from build123d import *

# Parameters (mm, degrees)
SKETCH2_R           = 0.26475865
BOSS_EXTRUDE1_DEPTH = 6.35


with BuildPart() as part:
    # Sketch1 → Revolve6 (revolve)
    with BuildSketch(Plane(origin=(0, 0, 0), x_dir=(0, 0, -1), z_dir=(1, 0, 0)), mode=Mode.PRIVATE) as revolve6_sk:
        with BuildLine():
            ThreePointArc((2.5, 0), (1.767766953, 1.767766953), (0, 2.5))
            Line((0, 2.5), (0, -7.09))
            Line((0, -7.09), (2.95, -7.09))
            Line((2.95, -7.09), (2.95, -6.09))
            Line((2.95, -6.09), (2.5, -6.09))
            Line((2.5, -6.09), (2.5, 0))
        make_face()
    revolve(revolve6_sk.sketch.rotate(Axis((0, 2.5, 0), (0, -1, 0)), 180), axis=Axis((0, 2.5, 0), (0, -1, 0)))

    # Sketch2 → Boss-Extrude1 (add)
    with BuildSketch(Plane.XZ.offset(7.09)):
        with Locations(Location((0, 1.283330706, 0), (0, 0, 90))):
            Circle(SKETCH2_R)
        with Locations(Location((0, -1.188269173, 0), (0, 0, 90))):
            Circle(SKETCH2_R)
    extrude(amount=BOSS_EXTRUDE1_DEPTH)


solid = part.part
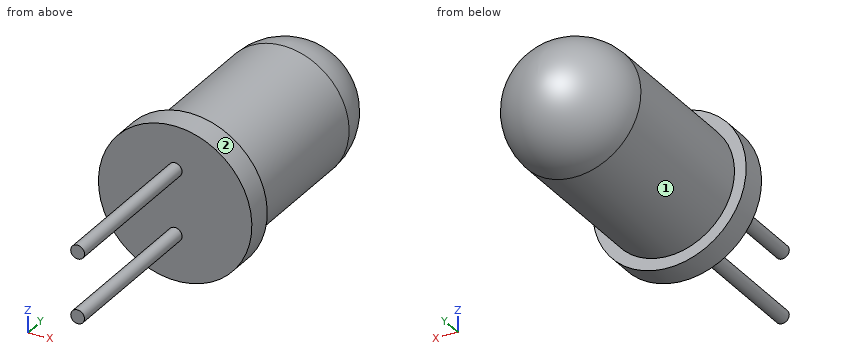
Geometry: final body of the model. Coordinates: model frame, mm. Face numbers are marked on the shaded views. A direction names the side the tool comes from. Coordinates: 2 decimals unless noted, no trailing zeros. Order: outer loops, then holes, each group sorted by start corner. A loop starts at its lowest first (then second) coordinate and runs counter-clockwise, first axis right, second up.
(1) Access query for the marked faces 1 and 2. Directions: +Z, -Z, +X, -X, +Y, -Y. A direction counts if a zero-diameter tool reaches every point of the face in a straight line with its end or side. Return the directions, or none.
(2) Material intervals for probe 1 along Y at (x, z) = (-1, -2.7); probe 2 along Z at (x, y) = (-1.7, -4.75); probe 3 along X at (y, z) = (0, -0.65), sorted ascending.
(3) Section query C-C (x = 0). Return the cut outline in (y, z).
(4) Section query D-D (y = -2). Return the cut outline in (x, z).
(5) First-contact query: pin 1 (2 mm diameter, centred on x = -2, z = 1, fed in from -Y); pin 2 (3 mm diameter, centred on x = 1, z = 0, fed in from +Y); pin 3 (3 mm diameter, centred on x = 1.5, y = 0, fed in from -Z). Flat tips, straight axial feed; report the tip coordinate or a pass-through.
(6) Section query B-B (y = -8.5). Return the cut outline in (x, z), plus the area to 3 significant figures.
(7) Section query A-A (z = 0). Return the cut outline in (x, y), plus the area to 3 significant figures.
Solution:
1. face 1: +Y
1. face 2: +Y, -Y
2. probe 1: y = -7.09 to -6.09
2. probe 2: z = -1.83 to 1.83
2. probe 3: x = -2.41 to 2.41
3. outline: (-13.44, -1.45) - (-7.09, -1.45) - (-7.09, -2.95) - (-6.09, -2.95) - (-6.09, -2.5) - (0, -2.5) arc R2.5 ccw to (0, 2.5) - (-6.09, 2.5) - (-6.09, 2.95) - (-7.09, 2.95) - (-7.09, 1.55) - (-13.44, 1.55) - (-13.44, 1.02) - (-7.09, 1.02) - (-7.09, -0.92) - (-13.44, -0.92) - close
4. outline: circle Ø5 at (0, 0)
5. pin 1: stops at y = -7.09
5. pin 2: stops at y = 2.5
5. pin 3: stops at z = -2.5
6. outline: circle Ø0.53 at (0, -1.19); circle Ø0.53 at (0, 1.28)
6. area: 0.440 mm2
7. outline: (-2.95, -7.09) - (2.95, -7.09) - (2.95, -6.09) - (2.5, -6.09) - (2.5, 0) arc R2.5 ccw to (-2.5, 0) - (-2.5, -6.09) - (-2.95, -6.09) - close
7. area: 46.2 mm2
